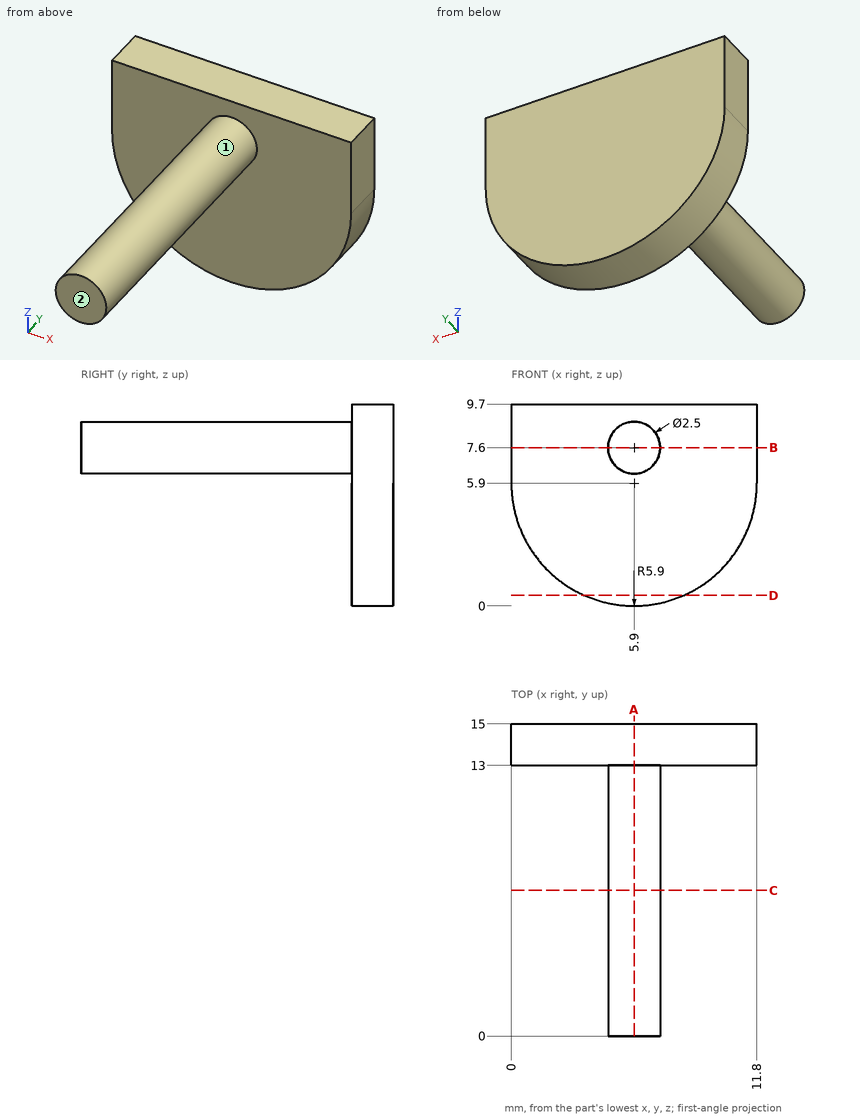
Here's the drawing with two shaded views (mm, measured from the low corner). I have some questions. A direction names the side the tool comes from. Give positions to 0.01 mm unless a question says otherwise; leave off trailing zeros. Write each loop counter-clockwise with the first axis right and the second up, starting at its lowest first coordinate (ties: lowest second). Pieces come first, ordered by that corner, then holes. Notation, with made-up numbers: (84, 83) -> (116, 83) arc R26 ccw to (116, 114) -> close; hole circle Ø6 at (29, 18). An arc over 180 degrees is marked (long way). One line per item, written item: value.
Q1. Which directions (+Z, -Z, +X, -X, +Y, -Y) give clear straight access to the entire face, cutting with the end or side of a thin tool? Please do the marked faces 1 and 2.
Results found:
face 1: -Y
face 2: +Z, -Z, +X, -X, -Y
Q2. Imagine slicing it at C-C on y = 7. Please give me the cut outline in (x, z).
Results found:
outline: circle Ø2.5 at (5.9, 7.6)
Q3. Imagine slicing it at B-B on z = 7.6. Please give me the cut outline in (x, y), and give its area (3 significant figures).
Results found:
outline: (0, 13) -> (4.65, 13) -> (4.65, 0) -> (7.15, 0) -> (7.15, 13) -> (11.8, 13) -> (11.8, 15) -> (0, 15) -> close
area: 56.1 mm^2
Q4. Please list where these lines run through material, in increasing order: line 1 (Y direction, x = 0.5, z = 7.5); line 2 (Z direction, x = 5.75, y = 14.5); line 3 (Z direction, x = 6, y = 12.75). Write a range as [from, to].
Results found:
line 1: y = [13, 15]
line 2: z = [0, 9.7]
line 3: z = [6.35, 8.85]
Q5. For P1, Ø1.5, axis at x = 10, z = 1.5, coming from the +Y side; P2, Ø1, axis at x = 9, y = 6, coming from the -Z side; P3, Ø4, axis at x = 5, z = 2.5, coming from the -Y side; P4, Ø6, axis at x = 3, y = 7.5, coming from the +Z side, each with a flat end and sliding along its axis, tell me the tip position at first contact or that it passes through.
Results found:
P1: stops at y = 15
P2: passes through
P3: stops at y = 13
P4: stops at z = 8.85
Q6. Imagine slicing it at D-D on z = 0.5. Please give me the cut outline in (x, y).
Results found:
outline: (3.52, 13) -> (8.28, 13) -> (8.28, 15) -> (3.52, 15) -> close
Q7. Imagine slicing it at A-A on x = 5.9. Please give me the cut outline in (y, z), and give its area (3 significant figures).
Results found:
outline: (0, 6.35) -> (13, 6.35) -> (13, 0) -> (15, 0) -> (15, 9.7) -> (13, 9.7) -> (13, 8.85) -> (0, 8.85) -> close
area: 51.9 mm^2
